Geometry: final body of the model. Coordinates: model frame, mm. A direction names the side the tool comes from. Give positions to 0.01 mm unless a question says otherwise; leave off trailing zeros. Order: outer loops, then holes, each group sorted by start corner. A loop starts at its lowest first (then second) coordinate and runs counter-clockwise, first axis right, second up. Notation, with made-up numbers: (67.5, 63.5) - (122.5, 63.5) arc R8 ccw to (122.5, 74.5) - close; hole circle Ø8 at (30, 64). An arc over 180 degrees is marked (long way). Put each result on its own line as item: value. Start each with the question number.
1. Set-up query: faces 5 (the flat face through (5.818, 41, 5)), 6 (the flat face through (2, -41, 5)), 7 (the flat face through (12, -38, 5)), 8 (the flat face through (31.725, -41, 5)). Return all of +Z, -Z, +X, -X, +Y, -Y with unobstructed straight access to the full face (end or side cutting, diameter ignored); none if empty.
2. Ray query, line 1 along X through (y, z) = (-42, 6.75); line 2 along Z through (x, y) = (31, -29.5); line 3 along Y through (x, z) = (7, 13.5). Return the intervals inside material, ascending. Write a range as from..to.
3. Section D-D on y = -29. Return the cut outline in (x, z).
4. Section B-B on x = 28.5. Return the cut outline in (y, z), plus the area to 3 significant figures.
5. Section A-A on y = 8. Return the cut outline in (x, z), plus the area to 4 significant figures.
6. First-contact query: P1, Ø1.5, axis at x = 16.5, z = 3.5, coming from the +Y side; P2, Ø12, axis at x = 7.5, y = -30.5, coming from the +Z side; P3, Ø1.5, axis at x = 10.5, z = 4, coming from the -Y side. Flat tips, straight axial feed; report the tip coordinate or a pass-through.
7. Section C-C on z = 16. Return the cut outline in (x, y), plus the area to 3 significant figures.
8. Mould query, pull axis Y, two halves, no side actions, for faces 1 (the flat face through (0, -47, 1)), 2 (the flat face through (10, 12.7, 10)), 3 (the flat face through (26, 41, 7.3)), 4 (the flat face through (26, 43.22, 5)). Classes: pulls with the +Y half, pulls with the -Y half, needs draft (parallel to the pull), parting line crosses it, or undercut.
from build123d import *

# Parameters (mm, degrees)
SKETCH2_W           = 70
SKETCH2_H           = 94
BOSS_EXTRUDE1_DEPTH = 2.3
SKETCH3_W           = 51.5
SKETCH3_H           = 12.7
BOSS_EXTRUDE2_DEPTH = 15
SKETCH4_W           = 12
SKETCH4_H           = 5.220497566
BOSS_EXTRUDE3_DEPTH = 5


with BuildPart() as part:
    # Sketch2 → Boss-Extrude1 (new body)
    with BuildSketch(Plane.XY):
        Rectangle(SKETCH2_W, SKETCH2_H)
    extrude(amount=BOSS_EXTRUDE1_DEPTH)

    # Sketch3 → Boss-Extrude2 (add)
    with BuildSketch(Plane.XY.offset(2.3)):
        with Locations((9.25, 6.35)):
            Rectangle(SKETCH3_W, SKETCH3_H)
        with Locations((9.25, -6.35)):
            Rectangle(SKETCH3_W, SKETCH3_H)
        Polygon((35, 12.7), (35, 0), (35, -12.7), (36, -12.7), (36, 12.7), align=None)
    extrude(amount=BOSS_EXTRUDE2_DEPTH)

    # Sketch4 → Boss-Extrude3 (add)
    with BuildSketch(Plane.XY.offset(2.3)):
        with Locations((-4, 40.610248783)):
            Rectangle(SKETCH4_W, SKETCH4_H)
        with Locations((11.818181083, 40.610248783)):
            Rectangle(SKETCH4_W, SKETCH4_H)
        with Locations((25.725310397, 40.610248783)):
            Rectangle(SKETCH4_W, SKETCH4_H)
        with Locations((-4, -40.610248783)):
            Rectangle(SKETCH4_W, SKETCH4_H)
        with Locations((11.818181083, -40.610248783)):
            Rectangle(SKETCH4_W, SKETCH4_H)
        with Locations((25.725310397, -40.610248783)):
            Rectangle(SKETCH4_W, SKETCH4_H)
    extrude(amount=BOSS_EXTRUDE3_DEPTH)


solid = part.part
Resolved:
1. face 5: +Z, +Y
1. face 6: +Z, -Y
1. face 7: +Z, +X, -X
1. face 8: +Z, +X, -Y
2. line 1: -10..2, 5.82..17.82, 19.73..31.73
2. line 2: 0..2.3
2. line 3: -12.7..12.7
3. outline: (-35, 0) - (35, 0) - (35, 2.3) - (-35, 2.3) - close
4. outline: (-47, 0) - (47, 0) - (47, 2.3) - (43.22, 2.3) - (43.22, 7.3) - (38, 7.3) - (38, 2.3) - (12.7, 2.3) - (12.7, 17.3) - (-12.7, 17.3) - (-12.7, 2.3) - (-38, 2.3) - (-38, 7.3) - (-43.22, 7.3) - (-43.22, 2.3) - (-47, 2.3) - close
4. area: 649 mm^2
5. outline: (-35, 0) - (35, 0) - (35, 2.3) - (36, 2.3) - (36, 17.3) - (-16.5, 17.3) - (-16.5, 2.3) - (-35, 2.3) - close
5. area: 948.5 mm^2
6. P1: y = 43.22
6. P2: z = 2.3
6. P3: y = -43.22
7. outline: (-16.5, -12.7) - (36, -12.7) - (36, 12.7) - (-16.5, 12.7) - close
7. area: 1,330 mm^2
8. face 1: pulls with the -Y half
8. face 2: undercut
8. face 3: needs draft
8. face 4: pulls with the +Y half
